The listing builds one solid part. Answer for the finished solid, in the listing's coordinates (mm). A direction names the side the tool comes from. Coordinates: 2 decimals unless noted, no trailing zeros. Write each loop counter-clockwise with the first axis right and the second up, starting at its lowest first coordinate (ties: lowest second). Pieces come first, ordered by that corner, then holes.
from build123d import *

# Parameters (mm, degrees)
ESQUISSE1_W                  = 30
ESQUISSE1_H                  = 30
BOSS_EXTRU_1_DEPTH           = 5
ENL_V_MAT_EXTRU_1_DEPTH      = 43.720018727
ENL_V_MAT_EXTRU_1_DEPTH_BACK = 43.720018727
ESQUISSE2_R                  = 5
ENL_V_MAT_EXTRU_2_DEPTH      = 43.720018727
ENL_V_MAT_EXTRU_2_DEPTH_BACK = 43.720018727
ESQUISSE3_W                  = 15
ESQUISSE3_H                  = 10
CONG_1_R                     = 2


with BuildPart() as part:
    # Esquisse1 → Boss.-Extru.1 (new body)
    with BuildSketch(Plane.XY):
        with Locations((15, 15)):
            Rectangle(ESQUISSE1_W, ESQUISSE1_H)
    extrude(amount=BOSS_EXTRU_1_DEPTH)

    # Esquisse2 → Enlèv. mat.-Extru.1 (cut, two sides: drawn at the far end of the back side and taken through both)
    with BuildSketch(Plane.XY.offset(5).offset(-ENL_V_MAT_EXTRU_1_DEPTH_BACK)):
        with Locations((15, 15)):
            Circle(ESQUISSE2_R)
    extrude(amount=ENL_V_MAT_EXTRU_1_DEPTH + ENL_V_MAT_EXTRU_1_DEPTH_BACK, mode=Mode.SUBTRACT)

    # Esquisse3 → Enlèv. mat.-Extru.2 (cut, two sides: drawn at the far end of the back side and taken through both)
    with BuildSketch(Plane.XY.offset(5).offset(-ENL_V_MAT_EXTRU_2_DEPTH_BACK)):
        with Locations((22.5, 15)):
            Rectangle(ESQUISSE3_W, ESQUISSE3_H)
    extrude(amount=ENL_V_MAT_EXTRU_2_DEPTH + ENL_V_MAT_EXTRU_2_DEPTH_BACK, mode=Mode.SUBTRACT)

    # Congé1
    cong_1_edges = [part.edges().sort_by_distance(p)[0] for p in [
        (30, 10, 2.5),
        (30, 20, 2.5),
        (30, 30, 2.5),
        (30, 0, 2.5),
        (0, 0, 2.5),
        (0, 30, 2.5),
    ]]
    fillet(cong_1_edges, radius=CONG_1_R)


solid = part.part
Q1. The part is cut by section B-B, the plane y = 12. Write down the section's boundary in (x, z), then the cut area to 3 significant figures.
Answers below:
outline: (0, 0) - (11, 0) - (11, 5) - (0, 5) - close
area: 55.0 mm2
Q2. The part is cut by section C-C, the plane y = 15. Write down the section's boundary in (x, z).
Answers below:
outline: (0, 0) - (10, 0) - (10, 5) - (0, 5) - close
Q3. Find the intervals of material crossed by probe 1 along Y at (x, z) = (25, 0.7); probe 2 along Y at (x, z) = (13.5, 2.05); probe 3 along Y at (x, z) = (1.5, 3.05), in increasing order.
Answers below:
probe 1: y = 0 to 10, 20 to 30
probe 2: y = 0 to 10.23, 19.77 to 30
probe 3: y = 0.06 to 29.94
Q4. The part is cut by section A-A, the plane z = 1.3. Write down the section's boundary in (x, y).
Answers below:
outline: (0, 2) arc R2 ccw to (2, 0) - (28, 0) arc R2 ccw to (30, 2) - (30, 8) arc R2 ccw to (28, 10) - (15, 10) arc R5 cw to (15, 20) - (28, 20) arc R2 ccw to (30, 22) - (30, 28) arc R2 ccw to (28, 30) - (2, 30) arc R2 ccw to (0, 28) - close
Q5. Which of the six approach directions +Z, -Z, +X, -X, +Y, -Y give full straight-line access (tool end or side, diameter ignored) to faces 5 (the face through (29.43, 20.6, 2.54)), 6 (the face through (0.57, 0.6, 2.54))?
Answers below:
face 5: +Z, -Z, +X
face 6: +Z, -Z, -X, -Y
Q6. Determine the mould class of faces 1 (the face through (21, 10, 2)), 2 (the face through (29.4, 0.57, 2.54)), 3 (the face through (11, 19, 5)), 4 (the face through (10, 15, 2)) for opening direction Y: released by +Y, released by -Y, zero draft, split by the parting line, or undercut.
Answers below:
face 1: undercut
face 2: released by -Y
face 3: zero draft
face 4: undercut
